Check sheet for the drawn part. Datum: minimum x, y, z corner. Units: mm. A direction names the side the tool comes from. Round coordinates to 2 decimals unless told otherwise and drop trailing zeros. Write each loop counter-clockwise with the first axis right and the second up, starting at its lowest first coordinate (ties: lowest second). Pieces come first, ordered by that corner, then holes. Notation, with made-up numbers: (10.5, 72) - (64.5, 72) arc R16 ccw to (64.5, 99) - close; hole circle Ø2 at (77, 60.25). An arc over 180 degrees is marked (long way). Answer as a JSON object with one key per item and string values.
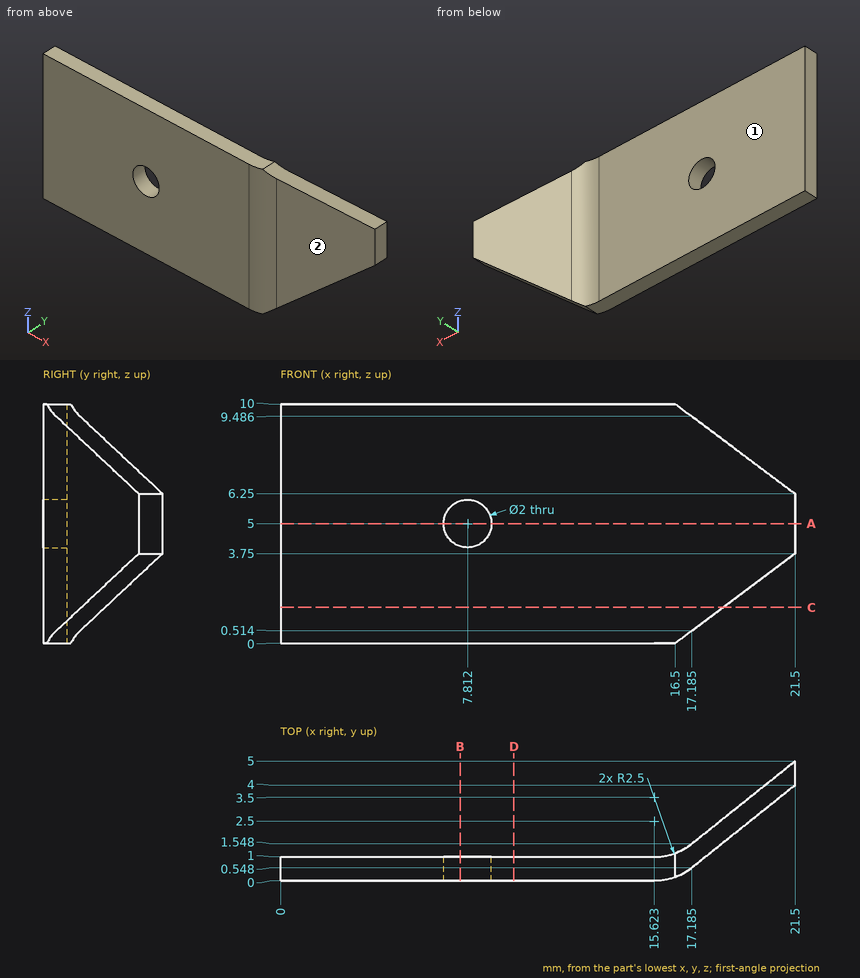
Q1. Gauge pin test, flat ends, axial feed: P1, Ø5, axis at x = 9, z = 3, coming from the +Y side; P2, Ø1.2, axis at x = 7.81, z = 5, coming from the +Y side; P3, Ø1.5, axis at x = 17.5, z = 6, coming from the -Y side. Record the tip position at first contact, or that the pin passes through.
Geometry check:
{"P1": "stops at y = 1", "P2": "passes through", "P3": "stops at y = 0.27"}
Q2. Section check D-D, the plane x = 9.75. Record the cut outline in (y, z).
Geometry check:
{"outline": "(0, 0) - (1, 0) - (1, 10) - (0, 10) - close"}
Q3. Section check A-A, the plane z = 5. Record the cut outline in (x, y) (1 decimal).
Geometry check:
{"outline": "(0, 0) - (6.8, 0) - (6.8, 1) - (0, 1) - close; (8.8, 0) - (15.6, 0) arc R2.5 ccw to (17.2, 0.5) - (21.5, 4) - (21.5, 5) - (17.2, 1.5) arc R2.5 cw to (15.6, 1) - (8.8, 1) - close"}
Q4. Set-up check for the marked faces 1 and 2: record each of +Z, -Z, +X, -X, +Y, -Y from which the full face is reachable in a straight line by a thin tool's end or side.
Geometry check:
{"face 1": "+Z, -Z, -X, +Y", "face 2": "+Z, -Z, +X, -Y"}
Q5. Section check C-C, the plane z = 1.5. Record the cut outline in (x, y) (1 decimal), then the cut area to 3 significant figures.
Geometry check:
{"outline": "(0, 0) - (15.6, 0) arc R2.5 ccw to (17.2, 0.5) - (18.5, 1.6) - (18.5, 2.6) - (17.2, 1.5) arc R2.5 cw to (15.6, 1) - (0, 1) - close", "area": "18.5 mm2"}
Q6. Section check B-B, the plane x = 7.5. Record the cut outline in (y, z).
Geometry check:
{"outline": "(0, 0) - (1, 0) - (1, 4.05) - (0, 4.05) - close; (0, 5.95) - (1, 5.95) - (1, 10) - (0, 10) - close"}
Q7. Material ranges on line 1 along Y through (x, z) = (8, 7.75); line 2 along X through (y, z) = (0.6, 5); line 3 along X through (y, z) = (0.3, 5) (1 decimal), recorded low to high. Write a range as [from, to].
Geometry check:
{"line 1": "y = [0, 1]", "line 2": "x = [0, 6.81], [8.81, 17.25]", "line 3": "x = [0, 6.8], [8.8, 16.8]"}
